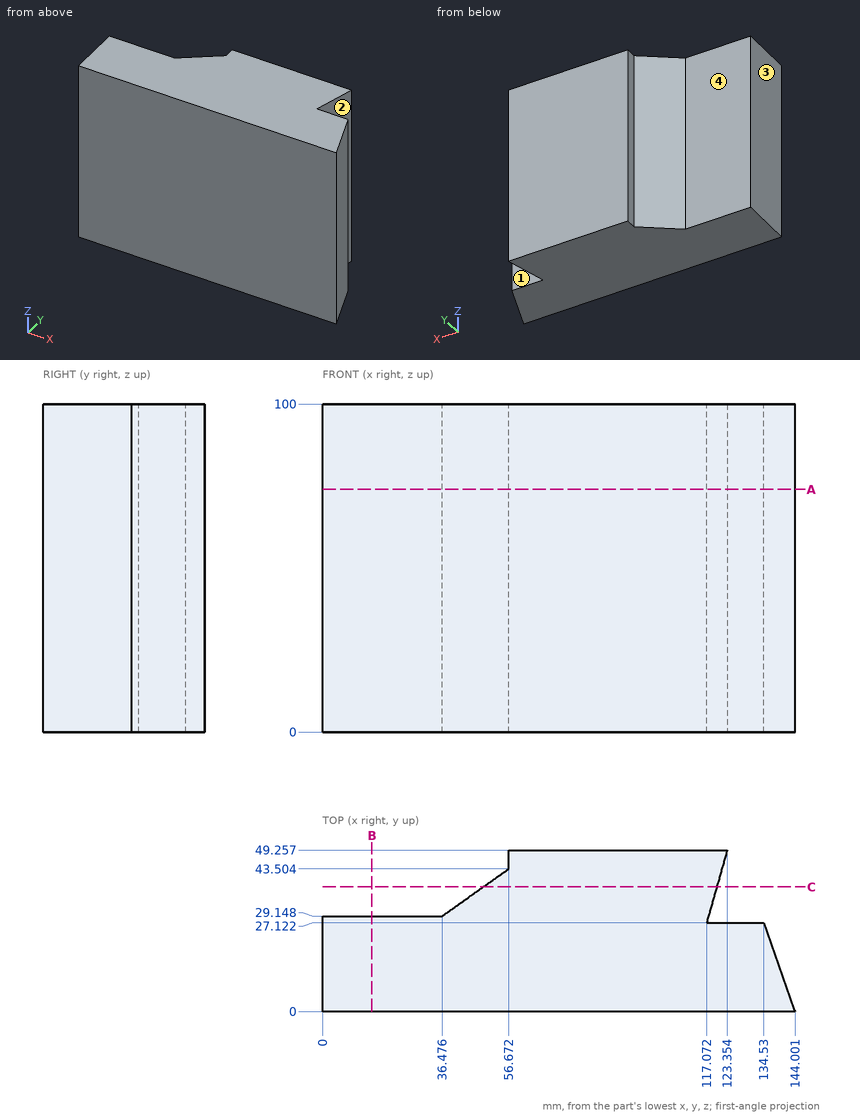
Input: dimensioned drawing with shaded views. Units: mm. Origin: part minimum x, y, z. Give positions to 0.01 mm unless a question says otherwise; leave off trailing zeros. Write each loop counter-clockwise with the first axis right and the second up, starting at its lowest first coordinate (ties: lowest second). Pieces come first, ordered by that corner, then holes.
1. Material intervals for line 1 along Y through (x, z) = (17, 69.5); line 2 along X through (y, z) = (37, 47) (1 decimal); line 3 along Y through (x, z) = (130, 77.5), sorted ascending.
2. Section query C-C (y = 38). Return the cut outline in (x, z), then the cut area to 3 significant figures.
3. Section query B-B (x = 15). Return the cut outline in (y, z).
4. Section query A-A (z = 74). Return the cut outline in (x, y) (1 decimal).
5. Pull-direction query (Y, two-part tool) for the marked faces 1, 2, 3 and 4; classes: +Y half, -Y half, draft (parallel to the pull), parting line (faces both ways), or undercut.
6. First-contact query: pin 1 (6.5 mm diameter, centred on y = 46.5, z = 26, fed in from -X) (1 decimal); pin 2 (12 mm diameter, centred on x = 15, z = 15.5, fed in from +Y); pin 3 (1.5 mm diameter, centred on y = 41.5, z = 61.5, fed in from +X) (1 decimal). Flat tips, straight axial feed; report the tip coordinate or a pass-through.
Output values:
1. line 1: y = 0 to 29.15
1. line 2: x = 47.5 to 119.9
1. line 3: y = 0 to 27.12
2. outline: (48.93, 0) - (120.16, 0) - (120.16, 100) - (48.93, 100) - close
2. area: 7,120 mm2
3. outline: (0, 0) - (29.15, 0) - (29.15, 100) - (0, 100) - close
4. outline: (0, 0) - (144, 0) - (134.5, 27.1) - (117.1, 27.1) - (123.4, 49.3) - (56.7, 49.3) - (56.7, 43.5) - (36.5, 29.1) - (0, 29.1) - close
5. face 1: undercut
5. face 2: undercut
5. face 3: draft
5. face 4: +Y half
6. pin 1: stops at x = 56.3
6. pin 2: stops at y = 29.15
6. pin 3: stops at x = 121.4
